CAD build for the part. Positions are in the model's coordinates, mm. A direction names the side the tool comes from. Round coordinates to 2 decimals unless told otherwise and drop trailing zeros. Loops run counter-clockwise (first coordinate to the right, second up) from the corner with the lowest first, then second, coordinate; pieces in that order, holes last. Notation, with made-up numbers: M 73.25,-18 L 100.25,-18 A10 cw 100.25,-6 Z; hole C 6.25,37.5 d10. An arc over 180 degrees is marked long. Use a Markdown table: item, result. Add a question column.
(1) Band-saw the part on A-A, the plane x = 0. Write the cut outline in (y, z).
(2) Wall check: L1, parallel to Z at x = 0, y = 3.25; L2, parallel to Z at x = 34, y = 0.5; L3, parallel to Z at x = 45, y = 1.75. Give the ranges that are in metal, low to high.
(3) Which spindle directions (+Z, -Z, +X, -X, +Y, -Y) get a long thin tool onto all of the face, cutting with end or side? Do faces 1 (the face through (-35.635, 3.219, 61.722)), 2 (the face through (-71, 3.22, -6.21)), 3 (the face through (71, 3.22, 6.21)). Say none if no direction does.
(4) Band-saw the part on B-B, the plane z = 52. Write the cut outline in (x, y).
(5) Two-plate mould, pull along Z, no slides. Class faces 4 (the face through (-67.35, 3.13, 35.64)), 5 (the face through (10.8, 3.13, 0.99)), 6 (the face through (-30.53, 3.22, -58.74)), 7 (the face through (-64.54, 3.13, -40.51)): released by +Z, released by -Z, zero draft, split by the parting line, or undercut.
(6) Flat gauge pins, fed straight in: P1, Ø3, axis at x = 55.5, y = 3, coming from the +Z side; P2, Ø2, axis at y = 4, z = -57.5, coming from the +X side; P3, Ø3.5, axis at x = -8.89, z = 0, coming from the +Y side; P4, Ø1, axis at y = 3, z = -15, coming from the -X side. Where does each tip first touch, or does it go through?
(7) Band-saw the part on D-D, the plane y = 1.25. Give the number of separate pieces and of enclosed holes in the cut face, and give its area (3 significant figures).
(8) Band-saw the part on C-C, the plane z = 36.5. Write the cut outline in (x, y).
Autodesk Inventor part; units mm, degrees
ref_plane "YZ Plane" through (0, 0, 0) normal (1, 0, 0) x (0, 1, 0)
ref_plane "XZ Plane" through (0, 0, 0) normal (0, 1, 0) x (-1, 0, 0)
ref_plane "XY Plane" through (0, 0, 0) normal (0, 0, 1) x (1, 0, 0)
sketch "Sketch1" plane through (0, 0, 0) normal (0, 1, 0) x (-1, 0, 0)
  circle A0 centre (0, -48.85) radius 21
  line L0 (0, -48.85) -> (0, 0) construction
  circle A1 centre (42.3053, -24.425) radius 21
  circle A2 centre (42.3053, 24.425) radius 21
  circle A3 centre (0, 48.85) radius 21
  circle A4 centre (-42.3053, 24.425) radius 21
  circle A5 centre (-42.3053, -24.425) radius 21
  circle A6 centre (0, 0) radius 76.2
  circle A7 centre (0, 0) radius 5.08
  dimension "d0" = 42
  dimension "d2" = 48.85
  dimension "d5" = 360
  dimension "d7" = 152.4
  dimension "d8" = 10.16
extrude "Extrusion1" add sketch "Sketch1" along normal blind 6.35
sketch "Sketch2" plane through (0, 6.35, 0) normal (0, 1, 0) x (1, 0, 0)
  circle A0 centre (0, 0) radius 5.08
  line L0 (-8.89, 0) -> (8.89, 0) construction
  dimension "d11" = 17.78
hole "Hole1" at (-8.89, 6.35, 0) at (8.89, 6.35, 0) direction (0, -1, 0) diameter 4.3053 end through all
sketch "Sketch3" plane through (0, 6.35, 0) normal (0, 1, 0) x (1, 0, 0)
  circle A0 centre (-8.89, 0) radius 2.1526
  circle A1 centre (0, 0) radius 5.08
  circle A2 centre (0, 0) radius 76.2
  line L0 (0, 0) -> (-8.89, 0) construction
  line L1 (-43.1, 74.6514) -> (-33.1, 57.3309)
  arc A3 (-36.4297, 78.1237) -> (-43.1, 74.6514) centre (0, 0) ccw
  arc A4 (-27.9773, 59.9976) -> (-33.1, 57.3309) centre (0, 0) ccw
  line L2 (-36.4297, 78.1237) -> (-27.9773, 59.9976)
  point P0 (-38.1, 65.9911)
  dimension "d30" = 60
  dimension "d35" = 20
  dimension "d37" = 20
  dimension "d38" = 65
extrude "Extrusion2" cut sketch "Sketch3" against normal through all contours L2 A4 L1 A2 | A2 L1 A3 L2 picked at (-32.0375, 65.438)
pattern_circular "Circular Pattern1" count 6 over 360 about axis through (0, -10, 0) along (0, 1, 0) of "Extrusion2"
equation "\"d37\" = d35"
properties part number "carousel-rev2"
Return value:
| question | item | result |
|---|---|---|
| 1 | outline | M 0,-76.2 L 6.35,-76.2 L 6.35,-69.85 L 0,-69.85 Z; M 0,-27.85 L 6.35,-27.85 L 6.35,-5.08 L 0,-5.08 Z; M 0,5.08 L 6.35,5.08 L 6.35,27.85 L 0,27.85 Z; M 0,69.85 L 6.35,69.85 L 6.35,76.2 L 0,76.2 Z |
| 2 | L1 | -76.2 to -69.85, -27.85 to -5.08, 5.08 to 27.85, 69.85 to 76.2 |
| 2 | L2 | -68.19 to -58.89, -56.8 to -43.71, -5.14 to 5.14, 43.71 to 58.89 |
| 2 | L3 | -61.49 to -45.25, -3.6 to 3.6, 45.25 to 61.49 |
| 3 | face 1 | +Y, -Y |
| 3 | face 2 | -X, +Y, -Y |
| 3 | face 3 | +X, +Y, -Y |
| 4 | outline | M -55.7,0 L -20.76,0 L -20.76,6.35 L -55.7,6.35 Z; M 20.76,0 L 55.7,0 L 55.7,6.35 L 20.76,6.35 Z |
| 5 | face 4 | released by +Z |
| 5 | face 5 | undercut |
| 5 | face 6 | undercut |
| 5 | face 7 | released by -Z |
| 6 | P1 | z = 53.76 |
| 6 | P2 | x = 51.13 |
| 6 | P3 | through |
| 6 | P4 | x = -74.81 |
| 7 | separate pieces | 1 |
| 7 | enclosed holes | 9 |
| 7 | area | 9,450 mm^2 |
| 8 | outline | M -66.89,0 L -59.49,0 L -59.49,6.35 L -66.89,6.35 Z; M -25.12,0 L -16.98,0 L -16.98,6.35 L -25.12,6.35 Z; M 16.98,0 L 25.12,0 L 25.12,6.35 L 16.98,6.35 Z; M 59.49,0 L 66.89,0 L 66.89,6.35 L 59.49,6.35 Z |
